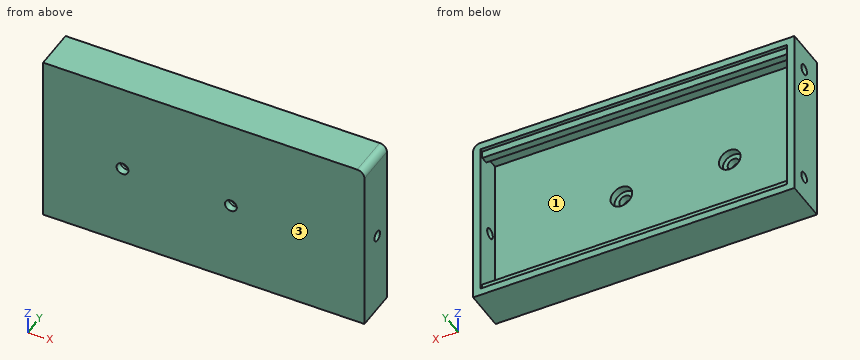
Autodesk Inventor part; units mm, degrees
ref_plane "YZ Plane" through (0, 0, 0) normal (1, 0, 0) x (0, 1, 0)
ref_plane "XZ Plane" through (0, 0, 0) normal (0, 1, 0) x (-1, 0, 0)
ref_plane "XY Plane" through (0, 0, 0) normal (0, 0, 1) x (1, 0, 0)
sketch "Sketch1" plane through (0, 0, 0) normal (0, 1, 0) x (-1, 0, 0)
  line L0 (0, 0) -> (0, -44)
  line L1 (0, -44) -> (85, -44)
  line L2 (85, -44) -> (85, 0)
  line L3 (85, 0) -> (0, 0)
  line L4 (0, 2) -> (85, 2)
  line L5 (85, 2) -> (87, 2)
  line L6 (87, 2) -> (87, -44)
  line L7 (87, -44) -> (87, -46)
  line L8 (87, -46) -> (0, -46)
  line L9 (0, -46) -> (-2, -46)
  line L10 (-2, -46) -> (-2, 2)
  line L11 (-2, 2) -> (0, 2)
  dimension "d0" = 44
  dimension "d1" = 85
  dimension "d2" = 2
  dimension "d3" = 2
  dimension "d4" = 2
  dimension "d5" = 2
extrude "Extrusion1" add sketch "Sketch1" along normal blind 4 contours L3 L2 L1 L0 | L4 L5 L6 L7 L8 L9 L10 L11
extrude "Extrusion2" add sketch "Sketch1" along normal blind 10.6
sketch "Sketch2" plane through (0, 10.6, 0) normal (0, 1, 0) x (1, 0, 0)
  line L0 (-87, -2) -> (-87, 46)
  line L1 (-87, -2) -> (-87, 46)
  line L2 (2, 46) -> (2, -2)
  line L3 (-87, 46) -> (2, 46)
  line L4 (2, 46) -> (2, -2)
  line L5 (2, -2) -> (-87, -2)
  line L6 (-85, 44) -> (-85, 0)
  line L7 (-85, 0) -> (-85, 44)
  line L8 (-85, 44) -> (0, 44)
  line L9 (0, 44) -> (0, 0)
  line L10 (0, 44) -> (0, 0)
  line L11 (0, 0) -> (-85, 0)
  line L12 (-85, 0) -> (-85, 2)
  line L13 (-85, 2) -> (0, 2)
  line L14 (-85, 44) -> (-85, 42)
  line L15 (-85, 42) -> (0, 42)
  dimension "d10" = 2
  dimension "d11" = 2
extrude "Extrusion3" add sketch "Sketch2" against normal blind 2 contours L8 L9 L15 L6 | L13 L9 L11 L6
extrude "Extrusion4" add sketch "Sketch2" along normal blind 1
fillet "Fillet1" radius 2 1 edges at (2, 5.8, 2)
sketch "Sketch3" plane through (2, 0, -46) normal (1, 0, 0) x (0, 0, -1)
  line L0 (0, 11.6) -> (-46, 11.6)
  line L1 (-23, 11.6) -> (-23, 6.6)
  circle A0 centre (-23, 6.6) radius 1.45
  point P0 (-46, 0)
  dimension "d17" = 5
  dimension "d18" = 2.9
extrude "Extrusion5" cut sketch "Sketch3" against normal blind 15
sketch "Sketch4" plane through (-87, 0, -46) normal (-1, 0, 0) x (0, 0, 1)
  line L0 (46, 11.6) -> (0, 11.6)
  line L1 (0, 11.6) -> (2, 11.6)
  line L2 (2, 11.6) -> (7, 11.6)
  line L3 (7, 11.6) -> (7, 6.6)
  line L4 (46, 0) -> (46, 11.6)
  line L5 (46, 11.6) -> (41, 11.6)
  line L6 (2, 11.6) -> (46, 11.6)
  line L7 (41, 11.6) -> (41, 6.6)
  circle A0 centre (7, 6.6) radius 1.45
  circle A1 centre (41, 6.6) radius 1.45
  dimension "d21" = 2
  dimension "d22" = 5
  dimension "d23" = 5
  dimension "d24" = 5
  dimension "d25" = 5
  dimension "d26" = 2.9
  dimension "d27" = 2.9
extrude "Extrusion6" cut sketch "Sketch4" against normal blind 15
sketch "Sketch5" plane through (0, 4, 0) normal (0, 1, 0) x (1, 0, 0)
  line L0 (-87, 46) -> (-87, 0)
  line L1 (-87, 23) -> (-65, 23)
  line L2 (-65, 23) -> (-35, 23)
  circle A0 centre (-65, 23) radius 1.65
  circle A1 centre (-35, 23) radius 1.65
  circle A2 centre (-35, 23) radius 3
  circle A3 centre (-65, 23) radius 3
  point P0 (0, 0)
  dimension "d30" = 22
  dimension "d31" = 30
  dimension "d32" = 3.3
  dimension "d33" = 3.3
  dimension "d34" = 6
  dimension "d35" = 6
extrude "Extrusion7" cut sketch "Sketch5" against normal blind 10 contours A1 | A0 L2 L1 | L1 L2 A0
extrude "Extrusion8" cut sketch "Sketch5" against normal blind 2 contours A3 L2 A0 L1 | A2 | L1 A0 L2 A3
properties part number "output"
Geometry: final body of the model. Coordinates: model frame, mm. Face numbers are marked on the shaded views. Give positions to 0.01 mm unless a question says otherwise; leave off trailing zeros. Order: outer loops, then holes, each group sorted by start corner. A loop starts at its lowest first (then second) coordinate and runs counter-clockwise, first axis right, second up. Notation, with made-up numbers: (-15.5, 18) - (8.5, 18) arc R26 ccw to (8.5, 36) - close; hole circle Ø3 at (-2.5, 64). An arc over 180 degrees is marked (long way). Use CSV: the item, a comma, the result in double quotes.
1. Contact query for flat-ended pins moving along their axis: pin 1 (2 mm diameter, centred on x = -46, z = -43.5, fed in from +Y); pin 2 (4 mm diameter, centred on x = -65, z = -23, fed in from +Y); pin 3 (5 mm diameter, centred on x = -26.5, z = -18.5, fed in from +Y). Output: stop coordinate, or through.
Answers below:
pin 1,"y = 11.6"
pin 2,"y = 2"
pin 3,"y = 4"
2. Section query A-A (x = -65). Output: boundary loops of the cut face in (y, z).
Answers below:
outline,"(0, -46) - (11.6, -46) - (11.6, -44) - (10.6, -44) - (10.6, -42) - (8.6, -42) - (8.6, -44) - (4, -44) - (4, -26) - (2, -26) - (2, -24.65) - (0, -24.65) - close; (0, -21.35) - (2, -21.35) - (2, -20) - (4, -20) - (4, 0) - (8.6, 0) - (8.6, -2) - (10.6, -2) - (10.6, 0) - (11.6, 0) - (11.6, 2) - (0, 2) - close"
3. Section query C-C (z = -23). Output: boundary loops of the cut face in (x, y).
Answers below:
outline,"(-87, 0) - (-66.65, 0) - (-66.65, 2) - (-68, 2) - (-68, 4) - (-85, 4) - (-85, 11.6) - (-87, 11.6) - close; (-63.35, 0) - (-36.65, 0) - (-36.65, 2) - (-38, 2) - (-38, 4) - (-62, 4) - (-62, 2) - (-63.35, 2) - close; (-33.35, 0) - (2, 0) - (2, 5.15) - (0, 5.15) - (0, 4) - (-32, 4) - (-32, 2) - (-33.35, 2) - close; (0, 8.05) - (2, 8.05) - (2, 11.6) - (0, 11.6) - close"
4. Material intervals for line 1 along X through (y, z) = (1.6, -23); line 2 along Z through (x, y) = (-85.8, 6.6); line 3 along Z through (x, y) = (-35, 0.8), sorted ascending. Write a range as from..to.
Answers below:
line 1,"-87..-66.65, -63.35..-36.65, -33.35..2"
line 2,"-46..-40.45, -37.55..-6.45, -3.55..2"
line 3,"-46..-24.65, -21.35..2"
5. Section query D-D (z = -39). Output: boundary loops of the cut face in (x, y).
Answers below:
outline,"(-87, 0) - (2, 0) - (2, 11.6) - (0, 11.6) - (0, 4) - (-85, 4) - (-85, 5.15) - (-87, 5.15) - close; (-87, 8.05) - (-85, 8.05) - (-85, 11.6) - (-87, 11.6) - close"
6. Mould query, pull axis X, two halves, no side actions, for the marked faces 1, 2 and 3. Classes: +X half, -X half, draft (parallel to the pull), parting line (faces both ways), or undercut.
Answers below:
face 1,"undercut"
face 2,"-X half"
face 3,"draft"
7. Section query B-B (y = 6.6). Output: boundary loops of the cut face in (x, z).
Answers below:
outline,"(-87, -46) - (2, -46) - (2, -24.45) - (0, -24.45) - (0, -44) - (-85, -44) - (-85, -40.45) - (-87, -40.45) - close; (-87, -37.55) - (-85, -37.55) - (-85, -6.45) - (-87, -6.45) - close; (-87, -3.55) - (-85, -3.55) - (-85, 0) - (0, 0) - (0, -21.55) - (2, -21.55) - (2, 0) arc R2 ccw to (0, 2) - (-87, 2) - close"
